Read the model definition and answer for the solid it produces. Units are mm, in the model's axes. A direction names the side the tool comes from. Coordinates: 2 decimals unless noted, no trailing zeros. Loops run counter-clockwise (first coordinate to the right, second up) from the corner with the lowest first, then second, coordinate; pieces in that order, holes last. Notation, with made-up numbers: (70, -22.75) -> (82, -22.75) arc R17 ccw to (82, -11.75) -> close; hole circle Ø6 at (27.25, 65.25). An arc over 180 degrees is marked (long way). Answer as CSV lines item,"result".
```python
from build123d import *

# Parameters (mm, degrees)
SALIENTE_EXTRUIR1_DEPTH = 5.02
CORTAR_EXTRUIR1_DEPTH   = 100
CROQUIS4_R              = 1.5
CORTAR_EXTRUIR2_DEPTH   = 10
CROQUIS5_R              = 3
CORTAR_EXTRUIR3_DEPTH   = 3.5
CORTAR_EXTRUIR4_DEPTH   = 100


with BuildPart() as part:
    # Croquis1 → Saliente-Extruir1 (new body)
    with BuildSketch(Plane(origin=(0, 0, 0), x_dir=(1, 0, 0), z_dir=(0, 1, 0))):
        Polygon((-46.116523403, 70), (-46.116523403, 100), (53.883476597, 100), (53.883476597, 70), (30.883476597, 70), (30.883476597, 40), (30.883476597, 0), (26.883476597, 0), (-19.116523403, 0), (-23.116523403, 0), (-23.116523403, 40), (-23.116523403, 70), align=None)
    extrude(amount=SALIENTE_EXTRUIR1_DEPTH)

    # Croquis2 → Cortar-Extruir1 (cut)
    with BuildSketch(Plane.ZY.offset(46.116523403)):
        Polygon((-100, 0), (-86.5, 5.02), (-100, 5.02), align=None)
    extrude(amount=-CORTAR_EXTRUIR1_DEPTH, mode=Mode.SUBTRACT)

    # Croquis4 → Cortar-Extruir2 (cut)
    with BuildSketch(Plane.XZ):
        with Locations(Location((3.883476597, -81, 0), (0, 0, 270))):
            Circle(CROQUIS4_R)
        with Locations(Location((24.383476597, -9.25, 0), (0, 0, 270))):
            Circle(CROQUIS4_R)
        with Locations(Location((-30.116523403, -81, 0), (0, 0, 270))):
            Circle(CROQUIS4_R)
        with Locations(Location((-13.116523403, -81, 0), (0, 0, 270))):
            Circle(CROQUIS4_R)
        with Locations(Location((24.383476597, -66.2, 0), (0, 0, 270))):
            Circle(CROQUIS4_R)
        with Locations(Location((24.383476597, -39.25, 0), (0, 0, 270))):
            Circle(CROQUIS4_R)
        with Locations(Location((-16.616523403, -9.25, 0), (0, 0, 270))):
            Circle(CROQUIS4_R)
        with Locations(Location((-16.616523403, -39.25, 0), (0, 0, 270))):
            Circle(CROQUIS4_R)
        with Locations(Location((-16.616523403, -66.2, 0), (0, 0, 270))):
            Circle(CROQUIS4_R)
        with Locations(Location((20.883476597, -81, 0), (0, 0, 270))):
            Circle(CROQUIS4_R)
        with Locations(Location((37.883476597, -81, 0), (0, 0, 270))):
            Circle(CROQUIS4_R)
    extrude(amount=-CORTAR_EXTRUIR2_DEPTH, mode=Mode.SUBTRACT)

    # Croquis5 → Cortar-Extruir3 (cut)
    with BuildSketch(Plane.XZ):
        with Locations(Location((24.383476597, -9.25, 0), (0, 0, 270))):
            Circle(CROQUIS5_R)
        with Locations(Location((24.383476597, -39.25, 0), (0, 0, 270))):
            Circle(CROQUIS5_R)
        with Locations(Location((24.383476597, -66.2, 0), (0, 0, 270))):
            Circle(CROQUIS5_R)
        with Locations(Location((-16.616523403, -66.2, 0), (0, 0, 90))):
            Circle(CROQUIS5_R)
        with Locations(Location((-16.616523403, -39.25, 0), (0, 0, 90))):
            Circle(CROQUIS5_R)
        with Locations(Location((-16.616523403, -9.25, 0), (0, 0, 90))):
            Circle(CROQUIS5_R)
        with Locations(Location((3.883476597, -81, 0), (0, 0, 270))):
            Circle(CROQUIS5_R)
        with Locations(Location((20.883476597, -81, 0), (0, 0, 270))):
            Circle(CROQUIS5_R)
        with Locations(Location((37.883476597, -81, 0), (0, 0, 270))):
            Circle(CROQUIS5_R)
        with Locations(Location((-30.116523403, -81, 0), (0, 0, 90))):
            Circle(CROQUIS5_R)
        with Locations(Location((-13.116523403, -81, 0), (0, 0, 90))):
            Circle(CROQUIS5_R)
    extrude(amount=-CORTAR_EXTRUIR3_DEPTH, mode=Mode.SUBTRACT)

    # Croquis6 → Cortar-Extruir4 (cut)
    with BuildSketch(Plane.ZY.offset(46.116523403)):
        Polygon((-100, 0), (-85, 0), (-96.250817152, 1.394140585), align=None)
    extrude(amount=-CORTAR_EXTRUIR4_DEPTH, mode=Mode.SUBTRACT)


solid = part.part
```
Q1. For a pull along Z with two mould halves and no side action, classify faces 1 (the face through (5, 5.02, -44)), 2 (the face through (-11.29, 1.73, -83.38)), 3 (the face through (-34, 2, -70)), 4 (the face through (3.2, 3.2, -91.4)) as pulls with the +Z half, pulls with the -Z half, needs draft (parallel to the pull), parting line crosses it, or undercut.
Results:
face 1,"needs draft"
face 2,"undercut"
face 3,"pulls with the +Z half"
face 4,"pulls with the -Z half"
Q2. Given pin 1 Ø2.5 at (x, z) = (24.38, -66.2) entering from +Y; pin 2 Ø5 at (x, z) = (-16.5, -66.5) entering from -Y; pin 3 Ø3 at (x, y) = (37.5, 0.5) entering from +Z; pin 4 Ø2 at (y, z) = (0.5, -49) entering from -X, each flat-ended and moving along its own axis, determine where each tip first touches the part or whether it passes through.
Results:
pin 1,"passes through"
pin 2,"stops at y = 3.5"
pin 3,"stops at z = -70"
pin 4,"stops at x = -23.12"
Q3. For faces 5 (the face through (-15.352, 4.249, -67.006)), 6 (the face through (30.883, 2, -35)), 7 (the face through (-28.29, 1.73, -83.38)), determine the directions among +Z, -Z, +X, -X, +Y, -Y from which every point of the face is accessible in a straight line to the end or side of a thin tool.
Results:
face 5,"+Y, -Y"
face 6,"+Z, +X, +Y, -Y"
face 7,"-Y"
Q4. A cutting plane is placed at A-A, the plane z = -39.25. Write down the section's boundary in (x, y), and give its area (3 significant figures).
Results:
outline,"(-23.12, 0) -> (-19.62, 0) -> (-19.62, 3.5) -> (-18.12, 3.5) -> (-18.12, 5.02) -> (-23.12, 5.02) -> close; (-15.12, 3.5) -> (-13.62, 3.5) -> (-13.62, 0) -> (21.38, 0) -> (21.38, 3.5) -> (22.88, 3.5) -> (22.88, 5.02) -> (-15.12, 5.02) -> close; (25.88, 3.5) -> (27.38, 3.5) -> (27.38, 0) -> (30.88, 0) -> (30.88, 5.02) -> (25.88, 5.02) -> close"
area,"220 mm²"
Q5. Find the intervals of material crossed by probe 1 along X at (y, z) = (4.3, -81); probe 2 along X at (y, z) = (2.35, -81); probe 3 along X at (y, z) = (1.75, -9.25), in increasing order. Write a range as [from, to].
Results:
probe 1,"x = [-46.12, -31.62], [-28.62, -14.62], [-11.62, 2.38], [5.38, 19.38], [22.38, 36.38], [39.38, 53.88]"
probe 2,"x = [-46.12, -33.12], [-27.12, -16.12], [-10.12, 0.88], [6.88, 17.88], [23.88, 34.88], [40.88, 53.88]"
probe 3,"x = [-23.12, -19.62], [-13.62, 21.38], [27.38, 30.88]"
Q6. A cutting plane is placed at C-C, the plane z = -81. Give the number of separate pieces and of enclosed holes in the cut face, and give its area (3 significant figures).
Results:
separate pieces,"6"
enclosed holes,"0"
area,"374 mm²"
Q7. A cutting plane is placed at B-B, the plane x = 12. Write down the section's boundary in (y, z).
Results:
outline,"(0, -85) -> (1.39, -96.25) -> (5.02, -86.5) -> (5.02, 0) -> (0, 0) -> close"
